```python
from build123d import *

# Parameters (mm, degrees)
HIERRO_ANGULAR_2_X_2_X_0_125_1_DEPTH = 50.8
CROQUIS3_R                           = 11.75
CROQUIS3_R_2                         = 2
CORTAR_EXTRUIR1_DEPTH                = 3.175
CROQUIS4_R                           = 2
CORTAR_EXTRUIR2_DEPTH                = 3.175


with BuildPart() as part:
    # Sketch1 → Hierro angular 2 X 2 X 0.125(1) (new body)
    with BuildSketch(Plane.YZ.offset(-25.4)):
        with BuildLine():
            Line((0, 0), (0, 50.8))
            Line((0, 50.8), (0.00508, 50.8))
            ThreePointArc((0.00508, 50.8), (2.246551928, 49.871551928), (3.175, 47.63008))
            Line((3.175, 47.63008), (3.175, 7.9375))
            ThreePointArc((3.175, 7.9375), (4.569903955, 4.569903955), (7.9375, 3.175))
            Line((7.9375, 3.175), (47.63008, 3.175))
            ThreePointArc((47.63008, 3.175), (49.871551928, 2.246551928), (50.8, 0.00508))
            Line((50.8, 0.00508), (50.8, 0))
            Line((50.8, 0), (0, 0))
        make_face()
    extrude(amount=HIERRO_ANGULAR_2_X_2_X_0_125_1_DEPTH)

    # Croquis3 → Cortar-Extruir1 (cut)
    with BuildSketch(Plane(origin=(0, 0, 0), x_dir=(-1, 0, 0), z_dir=(0, 0, -1))):
        with Locations((0, 25.4)):
            Circle(CROQUIS3_R)
        with Locations((-15.5, 40.9)):
            Circle(CROQUIS3_R_2)
        with Locations((15.5, 40.9)):
            Circle(CROQUIS3_R_2)
        with Locations((15.5, 9.9)):
            Circle(CROQUIS3_R_2)
        with Locations((-15.5, 9.9)):
            Circle(CROQUIS3_R_2)
    extrude(amount=-CORTAR_EXTRUIR1_DEPTH, mode=Mode.SUBTRACT)

    # Croquis4 → Cortar-Extruir2 (cut)
    with BuildSketch(Plane(origin=(0, 3.175, 0), x_dir=(1, 0, 0), z_dir=(0, 1, 0))):
        with Locations(Location((-17.5, -20.28379, 0), (0, 0, 270))):
            Circle(CROQUIS4_R)
        with Locations(Location((17.5, -20.28379, 0), (0, 0, 270))):
            Circle(CROQUIS4_R)
        with Locations(Location((17.5, -35.28379, 0), (0, 0, 270))):
            Circle(CROQUIS4_R)
        with Locations(Location((-17.5, -35.28379, 0), (0, 0, 270))):
            Circle(CROQUIS4_R)
        with Locations(Location((0, -20.28379, 0), (0, 0, 270))):
            Circle(CROQUIS4_R)
        with Locations(Location((0, -35.28379, 0), (0, 0, 270))):
            Circle(CROQUIS4_R)
    extrude(amount=-CORTAR_EXTRUIR2_DEPTH, mode=Mode.SUBTRACT)


solid = part.part
```
The model under review builds one solid part; all positions refer to its coordinate system, in mm. A direction names the side the tool comes from. Give positions to 0.01 mm unless a question says otherwise; leave off trailing zeros. Write each loop counter-clockwise with the first axis right and the second up, starting at its lowest first coordinate (ties: lowest second). Pieces come first, ordered by that corner, then holes. Notation, with made-up numbers: M 32,-40 L 74,-40 A19 cw 74,-14 Z; hole C 48.5,-40 d9. An arc over 180 degrees is marked long. Answer in a Markdown table with one row per item.
Item 1: Draft analysis for pull direction X (two halves, no side actions). For faces 1 (the face through (-6, 36, 3.175)), 2 (the face through (25.4, 14, 3)), 3 (the face through (-15.066, 38.948, 1.565)), state which applies: +X half, -X half, draft (parallel to the pull), parting line (faces both ways), or undercut.
Check sheet entries:
| item | result |
|---|---|
| face 1 | draft |
| face 2 | +X half |
| face 3 | undercut |
Item 2: Tool access review of faces 4 (the face through (-16.15, 1.61, 33.81)), 5 (the face through (0, 3.175, 28)): name each direction out of +Z, -Z, +X, -X, +Y, -Y from which nothing blocks a thin tool from reaching the whole face with its end or side.
Check sheet entries:
| item | result |
|---|---|
| face 4 | +Y, -Y |
| face 5 | +Z, +X, -X, +Y |
Item 3: Add section A-A on y = 16. Give the boundary of the cut face in (x, z) (3 decimals), plus the area to 3 significant figures.
Check sheet entries:
| item | result |
|---|---|
| outline | M -25.4,0 L -7.05,0 L -7.05,3.175 L -25.4,3.175 Z; M 7.05,0 L 25.4,0 L 25.4,3.175 L 7.05,3.175 Z |
| area | 117 mm2 |
Item 4: Add section B-B on x = 0. State how many separate pieces and enclosed holes the cut face has, plus the area to 3 significant figures.
Check sheet entries:
| item | result |
|---|---|
| separate pieces | 4 |
| enclosed holes | 0 |
| area | 213 mm2 |
Item 5: For line 1 along X through (y, z) = (40, 2); line 2 along X through (y, z) = (25, 1); line 3 along Y through (x, z) = (-15, 2), list the stretches that pass through material, from the lowest coordinate up.
Check sheet entries:
| item | result |
|---|---|
| line 1 | -25.4 to -17.29, -13.71 to 13.71, 17.29 to 25.4 |
| line 2 | -25.4 to -11.74, 11.74 to 25.4 |
| line 3 | 0 to 7.96, 11.84 to 38.96, 42.84 to 50.09 |
Item 6: For P1, Ø12, axis at x = -19, y = 22, coming from the -Z side; P2, Ø4, axis at x = -2, y = 8.5, coming from the +Z side; P3, Ø3, axis at x = 0, z = 36, coming from the +Y side (3 decimals); P4, Ø20, axis at x = -11, y = 34, coming from the +Z side (3 decimals), all flat-tipped, find the tip position at first contact; note any pin that passes through.
Check sheet entries:
| item | result |
|---|---|
| P1 | z = 0 |
| P2 | z = 3.4 |
| P3 | y = 3.175 |
| P4 | z = 3.175 |
Item 7: Add section C-C on y = 9.9. Give the boundary of the cut face in (x, z) (3 decimals).
Check sheet entries:
| item | result |
|---|---|
| outline | M -25.4,0 L -17.5,0 L -17.5,3.175 L -25.4,3.175 Z; M -13.5,0 L 13.5,0 L 13.5,3.175 L -13.5,3.175 Z; M 17.5,0 L 25.4,0 L 25.4,3.175 L 17.5,3.175 Z |
